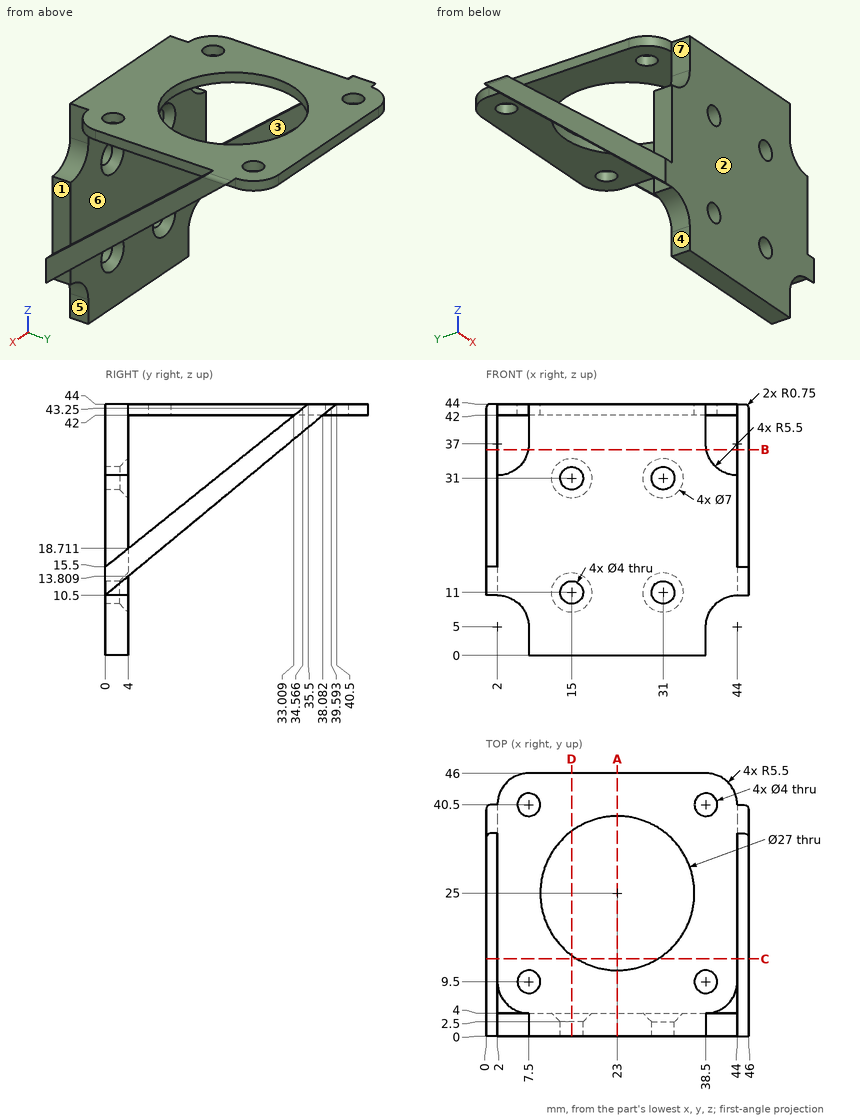
For this review, use the dimensioned drawing (mm, ordinates from the lowest corner) and the shaded views. A direction names the side the tool comes from. Give positions to 0.01 mm unless a question says otherwise; leave off trailing zeros. Order: outer loops, then holes, each group sorted by start corner. A loop starts at its lowest first (then second) coordinate and runs counter-clockwise, first axis right, second up.
1) Take a section at D-D (x = 15). Give the boundary of the cut face in (y, z) (1 decimal).
2) Take a section at B-B (z = 36). Give the boundary of the cut face in (x, y) (1 decimal).
3) Take a section at A-A (x = 23). Give the boundary of the cut face in (y, z), then the cut area to 3 significant figures.
4) The part is to be moulded in two halves that separate along X. For the marked faces 1, 2 and 3, say which applies: released by +X, released by -X, zero draft, split by the parting line, or undercut.
5) Insertion check: pin 1 (2 mm diameter, centred on y = 2, z = 40, fed in from -X); pin 2 (5 mm diameter, centred on x = 36.5, z = 18, fed in from +Y); pin 3 (1.6 mm diameter, centred on y = 26.5, z = 43.5, fed in from -X). Each pin has a flat end and moves straight along its axis. Give the tip position at first contact, or say it passes through.
6) Take a section at C-C (y = 13.5). Give the boundary of the cut face in (x, z).
7) Wall thickness on line 1 (X direction, y = 1.7, z = 31); line 2 (Y direction, x = 26, z = 17); line 3 (Z direction, x = 17.5, y = 12.5): over which ranges is each line inside the solid? List them lowest first.
8) For the marked faces 4, 5, 6 and 7, list the 3-axis set-ups (+Z, -Z, +X, -X, +Y, -Y) from which the entire face can be reached by the end or side of a thin tool; tool diameter is ignored.
Derived:
1. outline: (0, 0) - (4, 0) - (4, 7.5) - (2.5, 9) - (0, 9) - close; (0, 13) - (2.5, 13) - (4, 14.5) - (4, 27.5) - (2.5, 29) - (0, 29) - close; (0, 33) - (2.5, 33) - (4, 34.5) - (4, 42) - (14.1, 42) - (14.1, 44) - (0, 44) - close; (35.9, 42) - (46, 42) - (46, 44) - (35.9, 44) - close
2. outline: (0, 25.5) - (2, 25.5) - (2, 30.8) - (0, 30.8) - close; (7.4, 0) - (38.6, 0) - (38.6, 4) - (7.4, 4) - close; (44, 25.5) - (46, 25.5) - (46, 30.8) - (44, 30.8) - close
3. outline: (0, 0) - (4, 0) - (4, 42) - (11.5, 42) - (11.5, 44) - (0, 44) - close; (38.5, 42) - (46, 42) - (46, 44) - (38.5, 44) - close
3. area: 206 mm2
4. face 1: released by +X
4. face 2: zero draft
4. face 3: undercut
5. pin 1: stops at x = 7.5
5. pin 2: stops at y = 4
5. pin 3: stops at x = 2
6. outline: (0, 21.67) - (2, 21.67) - (2, 26.34) - (0, 26.34) - close; (2, 42) - (15.93, 42) - (15.93, 44) - (2, 44) - close; (30.07, 42) - (44, 42) - (44, 44) - (30.07, 44) - close; (44, 21.67) - (46, 21.67) - (46, 26.34) - (44, 26.34) - close
7. line 1: x = 2 to 13, 17 to 29, 33 to 44
7. line 2: y = 0 to 4
7. line 3: z = 42 to 44
8. face 4: -Z, -X, +Y, -Y
8. face 5: -Z, +X, +Y, -Y
8. face 6: -Z, +Y
8. face 7: +Z, -X, -Y
